Build history of the part. All positions in model axes, mm. Face numbers are marked on the shaded views. A direction names the side the tool comes from. Coordinates: 2 decimals unless noted, no trailing zeros. Loops run counter-clockwise (first coordinate to the right, second up) from the corner with the lowest first, then second, coordinate; pieces in that order, holes last.
(1) Two-plate mould, pull along X, no slides. Class the marked faces 1, 2, 3 and 4: pulls with the +X half, pulls with the -X half, needs draft (parallel to the pull), parting line crosses it, or undercut.
(2) Slice it at D-D (z = 2.25). Give the cut face in (x, y).
(3) Slice it at C-C (x = -2.1). Give the cut face in (y, z), and give its area (3 significant figures).
(4) Slice it at A-A (z = 0). Give the cut face in (x, y).
(5) Slice it at B-B (x = 0). Give the cut face in (y, z), and give its area (3 significant figures).
(6) Wall check: L1, parallel to Z at x = 0, y = -2.05; L2, parallel to Z at x = -0.25, y = -4.65; L3, parallel to X at y = -1.5, z = -0.2. Give the ranges that are in metal, low to high.
(7) Flat gauge pin, fed straight in: P1, Ø2, axis at x = 2, y = -2.5, coming from the -Z side. Where does the tip first touch, or does it go through?
(8) Tool access for the marked faces 5, 6, 7, 8 and 9: list every direction of +Z, -Z, +X, -X, +Y, -Y with a clear straight run to the whole face (end or side of a thin tool).
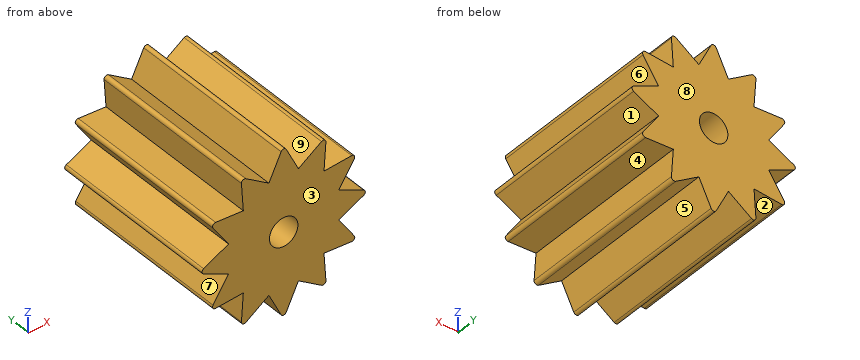
from build123d import *

# Parameters (mm, degrees)
F0_R     = 0.5
F1_DEPTH = 6
F2_DEPTH = 6
F3_R     = 0.1
F4_COUNT = 12


with BuildPart() as f1:
    # F0 (on Front) → F1 (new body)
    with BuildSketch(Plane.XZ):
        with BuildLine():
            ThreePointArc((-0.5233333333, 1.9303166119), (-1.2151817422, -1.588500341), (2, 0))
            ThreePointArc((2, 0), (1.588500341, 1.2151817422), (0.5233333333, 1.9303166119))
            ThreePointArc((0.5233333333, 1.9303166119), (0, 2), (-0.5233333333, 1.9303166119))
        make_face()
        Circle(F0_R, mode=Mode.SUBTRACT)
    extrude(amount=F1_DEPTH)



with BuildPart() as f2:
    # F0 (on Front) → F2 (new body)
    with BuildSketch(Plane.XZ):
        with BuildLine():
            ThreePointArc((-0.5233333333, 1.9303166119), (0, 2), (0.5233333333, 1.9303166119))
            Line((0.5233333333, 1.9303166119), (0, 3))
            Line((0, 3), (-0.5233333333, 1.9303166119))
        make_face()
    extrude(amount=F2_DEPTH)

    # F3
    f3_edges = [f2.edges().sort_by_distance(p)[0] for p in [
        (0, -3, 3),
    ]]
    fillet(f3_edges, radius=F3_R)


with BuildPart() as f1_1:
    add(f1.part)

    add(f2.part)  # F4 merges F2
    # F4: F2 ×12 about axis
    f4_axis = Axis((0, 0, 0), (0, -1, 0))
    for i in range(1, F4_COUNT):
        add(f2.part.rotate(f4_axis, i * 360 / F4_COUNT))


solid = f1_1.part
Response values:
1. face 1: pulls with the +X half
1. face 2: undercut
1. face 3: needs draft
1. face 4: undercut
2. outline: (-1.48, -6) - (-0.98, -6) - (-0.98, 0) - (-1.48, 0) - close; (-0.37, -6) - (0.37, -6) - (0.37, 0) - (-0.37, 0) - close; (0.98, -6) - (1.48, -6) - (1.48, 0) - (0.98, 0) - close
3. outline: (-6, -1.47) - (0, -1.47) - (0, -0.76) - (-6, -0.76) - close; (-6, -0.44) - (0, -0.44) - (0, 0.44) - (-6, 0.44) - close; (-6, 0.76) - (0, 0.76) - (0, 1.47) - (-6, 1.47) - close
3. area: 13.8 mm2
4. outline: (-2.87, -6) - (-0.5, -6) - (-0.5, 0) - (-2.87, 0) - close; (0.5, -6) - (2.87, -6) - (2.87, 0) - (0.5, 0) - close
5. outline: (-6, -2.87) - (0, -2.87) - (0, -0.5) - (-6, -0.5) - close; (-6, 0.5) - (0, 0.5) - (0, 2.87) - (-6, 2.87) - close
5. area: 28.5 mm2
6. L1: z = -2.87 to -0.5, 0.5 to 2.87
6. L2: z = -2.49 to -0.43, 0.43 to 2.49
6. L3: x = -2.59 to -0.46, 0.46 to 2.59
7. P1: stops at z = -2.5
8. face 5: -Z, +Y, -Y
8. face 6: +X, +Y, -Y
8. face 7: -X, +Y, -Y
8. face 8: +Z, -Z, +X, -X, +Y
8. face 9: +Z, +Y, -Y
